Check sheet for the modelled part. Datum: model origin and axes. Units: mm. A direction names the side the tool comes from. Coordinates: 2 decimals unless noted, no trailing zeros. Write each loop counter-clockwise with the first axis right and the second up, starting at its lowest first coordinate (ties: lowest second). Pieces come first, ordered by that corner, then holes. Notation, with made-up numbers: M -25,10.5 L 31,10.5 A15 ccw 31,15.5 Z; hole C 57,72.5 d5. An arc over 180 degrees is marked long. Answer as CSV lines item,"result". Start each with the question number.
1) Section check A-A (z = 25.5). Record the cut outline in (x, y).
2) Section check D-D (z = -40). Record the cut outline in (x, y).
3) Access from +Z, -Z, +X, -X, +Y, -Y to the whole of each face (thin tool, end or side, straight path). Record for faces 1 (the flat face through (43.461, 2.415, 33.158)), 2 (the flat face through (-43.399, 2.415, -33.122)), 3 (the flat face through (-6.985, 2, -54)), 4 (the flat face through (-6.985, 2, 54)), 5 (the flat face through (-44.77, 2.41, -25.74)).
4) Section check C-C (x = 0). Record the cut outline in (y, z).
5) Go/stop test with flat-tipped pins: pin 1 Ø5 at (x, z) = (-28, -7) entering from -Y; pin 2 Ø2.5 at (y, z) = (3, 53) entering from -X; pin 3 Ø1.4 at (x, y) = (1.5, 2) entering from +Z; pin 4 Ø1.5 at (x, y) = (36, 3) entering from +Z. Record where each tip stops, or that it passes through.
6) Material ranges on L1, parallel to Z at x = -2.5, y = 3.1; L2, parallel to X at y = 4, z = -1.5; L3, parallel to Z at x = -32.5, y = 4, recorded low to high. Write a range as [from, to].
7) Section check B-B (y = 3.65). Record the cut outline in (x, z) (3 decimals).
8) Draft check along Z on faces 6 (the flat face through (6.985, 2, -54)), 7 (the flat face through (50.38, 2.41, 21.02)), 8 (the flat face through (44.67, 2.41, 25.91)). Enter one of: +Z half, -Z half, draft (parallel to the pull), parting line (faces both ways), or undercut.
from build123d import *

# Parameters (mm, degrees)
SKETCH1_R                  = 57.15
BOSS_EXTRUDE1_DEPTH        = 4.7625
CUT_EXTRUDE1_REACH         = 82.963
CUT_EXTRUDE2_REACH         = 82.661
F_4_0_209_DIAMETER_HOLE1_D = 5.3086


with BuildPart() as part:
    # Sketch1 → Boss-Extrude1 (new body)
    with BuildSketch(Plane(origin=(0, 0, 0), x_dir=(1, 0, 0), z_dir=(0, 1, 0))):
        with Locations(Location((0, 0, 0), (0, 0, 90))):
            Circle(SKETCH1_R)
    extrude(amount=BOSS_EXTRUDE1_DEPTH)

    # Sketch2 → Cut-Extrude1 (cut, up to next)
    with BuildSketch(Plane(origin=(0, 4.7625, 0), x_dir=(1, 0, 0), z_dir=(0, 1, 0)), mode=Mode.PRIVATE) as cut_extrude1_sk1:
        with BuildLine():
            Line((-6.985, -51.641532728), (6.985, -51.641532728))
            Line((6.985, -51.641532728), (6.985, -56.721532728))
            ThreePointArc((6.985, -56.721532728), (0, -57.15), (-6.985, -56.721532728))
            Line((-6.985, -56.721532728), (-6.985, -51.641532728))
        make_face()
    cut_extrude1_tool1 = extrude(cut_extrude1_sk1.sketch, amount=-CUT_EXTRUDE1_REACH, mode=Mode.PRIVATE) & part.part
    # Sketch2 → Cut-Extrude1 (cut, up to next)
    with BuildSketch(Plane(origin=(0, 4.7625, 0), x_dir=(1, 0, 0), z_dir=(0, 1, 0)), mode=Mode.PRIVATE) as cut_extrude1_sk2:
        with BuildLine():
            Line((-6.985, 51.641532728), (-6.985, 56.721532728))
            ThreePointArc((-6.985, 56.721532728), (0, 57.15), (6.985, 56.721532728))
            Line((6.985, 56.721532728), (6.985, 51.641532728))
            Line((6.985, 51.641532728), (-6.985, 51.641532728))
        make_face()
    cut_extrude1_tool2 = extrude(cut_extrude1_sk2.sketch, amount=-CUT_EXTRUDE1_REACH, mode=Mode.PRIVATE) & part.part
    add(cut_extrude1_tool1.solids().sort_by_distance((0, 4.7625, 54.325982))[0], mode=Mode.SUBTRACT)
    add(cut_extrude1_tool2.solids().sort_by_distance((0, 4.7625, -54.325982))[0], mode=Mode.SUBTRACT)

    # Sketch3 → Cut-Extrude2 (cut, up to next)
    with BuildSketch(Plane(origin=(0, 4.7625, 0), x_dir=(1, 0, 0), z_dir=(0, 1, 0)), mode=Mode.PRIVATE) as cut_extrude2_sk1:
        with BuildLine():
            Line((41.230379233, -31.869953809), (48.215379233, -19.771578919))
            Line((48.215379233, -19.771578919), (52.614788284, -22.311578919))
            ThreePointArc((52.614788284, -22.311578919), (49.493351826, -28.575), (45.629788284, -34.409953809))
            Line((45.629788284, -34.409953809), (41.230379233, -31.869953809))
        make_face()
    cut_extrude2_tool1 = extrude(cut_extrude2_sk1.sketch, amount=-CUT_EXTRUDE2_REACH, mode=Mode.PRIVATE) & part.part
    # Sketch3 → Cut-Extrude2 (cut, up to next)
    with BuildSketch(Plane(origin=(0, 4.7625, 0), x_dir=(1, 0, 0), z_dir=(0, 1, 0)), mode=Mode.PRIVATE) as cut_extrude2_sk2:
        with BuildLine():
            Line((-41.230379233, 31.869953809), (-45.629788284, 34.409953809))
            ThreePointArc((-45.629788284, 34.409953809), (-49.493351826, 28.575), (-52.614788284, 22.311578919))
            Line((-52.614788284, 22.311578919), (-48.215379233, 19.771578919))
            Line((-48.215379233, 19.771578919), (-41.230379233, 31.869953809))
        make_face()
    cut_extrude2_tool2 = extrude(cut_extrude2_sk2.sketch, amount=-CUT_EXTRUDE2_REACH, mode=Mode.PRIVATE) & part.part
    add(cut_extrude2_tool1.solids().sort_by_distance((47.04768, 4.7625, 27.162991))[0], mode=Mode.SUBTRACT)
    add(cut_extrude2_tool2.solids().sort_by_distance((-47.04768, 4.7625, -27.162991))[0], mode=Mode.SUBTRACT)

    # #4 (0.209) Diameter Hole1 (through all)
    with Locations(Plane(origin=(16.002, 4.7625, -24.638), x_dir=(0, 0, 1), z_dir=(0, 1, 0))):
        with Locations((0, 0), (49.022, 0), (49.022, -32.004), (0, -32.004)):
            Hole(F_4_0_209_DIAMETER_HOLE1_D / 2)


solid = part.part
Results found:
1,outline,"M -51.15,0 L -18.41,0 L -18.41,4.76 L -51.15,4.76 Z; M -13.59,0 L 13.59,0 L 13.59,4.76 L -13.59,4.76 Z; M 18.41,0 L 44.91,0 L 44.91,4.76 L 18.41,4.76 Z"
2,outline,"M -40.82,0 L 40.82,0 L 40.82,4.76 L -40.82,4.76 Z"
3,face 1,"+X, +Y, -Y"
3,face 2,"-X, +Y, -Y"
3,face 3,"-Z, +Y, -Y"
3,face 4,"+Z, +Y, -Y"
3,face 5,"+Y, -Y"
4,outline,"M 0,-51.64 L 4.76,-51.64 L 4.76,51.64 L 0,51.64 Z"
5,pin 1,"stops at y = 0"
5,pin 2,"stops at x = -24.25"
5,pin 3,"stops at z = 51.64"
5,pin 4,"stops at z = 44.98"
6,L1,"z = [-51.64, 51.64]"
6,L2,"x = [-57.13, 57.13]"
6,L3,"z = [-47.01, 47.01]"
7,outline,"M -52.615,-22.312 L -48.215,-19.772 L -41.23,-31.87 L -45.63,-34.41 A57.15 ccw -6.985,-56.722 L -6.985,-51.642 L 6.985,-51.642 L 6.985,-56.722 A57.15 ccw 52.615,22.312 L 48.215,19.772 L 41.23,31.87 L 45.63,34.41 A57.15 ccw 6.985,56.722 L 6.985,51.642 L -6.985,51.642 L -6.985,56.722 A57.15 ccw Z; hole C -16.002,-24.638 d5.309; hole C -16.002,24.384 d5.309; hole C 16.002,-24.638 d5.309; hole C 16.002,24.384 d5.309"
8,face 6,"draft"
8,face 7,"+Z half"
8,face 8,"undercut"
